from build123d import *

# Parameters (mm, degrees)
ESQUISSE1_R             = 1
BOSS_EXTRU_1_DEPTH      = 10
ESQUISSE2_W             = 4
ESQUISSE2_H             = 7.5
ESQUISSE2_H_2           = 4.5
ENL_V_MAT_EXTRU_1_DEPTH = 15


with BuildPart() as part:
    # Esquisse1 → Boss.-Extru.1 (new body)
    with BuildSketch(Plane.XY):
        with BuildLine():
            ThreePointArc((-77.855878935, 59.113903977), (-67.897166599, 55.463691844), (-64.246954466, 65.422404179))
            Line((-64.246954466, 65.422404179), (-73.709704769, 85.835790883))
            Line((-73.709704769, 85.835790883), (-75.524228032, 84.994657522))
            Line((-75.524228032, 84.994657522), (-70.47742787, 74.107517947))
            Line((-70.47742787, 74.107517947), (-74.106474395, 72.425251227))
            Line((-74.106474395, 72.425251227), (-79.153274557, 83.312390802))
            Line((-79.153274557, 83.312390802), (-81.875059451, 82.050690761))
            Line((-81.875059451, 82.050690761), (-76.828259289, 71.163551186))
            Line((-76.828259289, 71.163551186), (-80.457305814, 69.481284466))
            Line((-80.457305814, 69.481284466), (-85.504105976, 80.368424041))
            Line((-85.504105976, 80.368424041), (-87.318629238, 79.52729068))
            Line((-87.318629238, 79.52729068), (-77.855878935, 59.113903977))
        make_face()
        with Locations((-71.0514167, 62.268154078)):
            Circle(ESQUISSE1_R, mode=Mode.SUBTRACT)
    extrude(amount=BOSS_EXTRU_1_DEPTH)

    # Esquisse2 → Enlèv. mat.-Extru.1 (cut)
    with BuildSketch(Plane(origin=(-41.529278226, -19.251151014, 0), x_dir=(0, 0, 1), z_dir=(-0.9072616312569987, -0.42056668014583576, 0))):
        with BuildLine():
            Line((5, 108.875365486), (0, 108.875365486))
            Line((0, 108.875365486), (0, 103.875365486))
            ThreePointArc((0, 103.875365486), (1.464466094, 107.410899392), (5, 108.875365486))
        make_face()
        with BuildLine():
            Line((10, 108.875365486), (5, 108.875365486))
            ThreePointArc((5, 108.875365486), (8.535533906, 107.410899392), (10, 103.875365486))
            Line((10, 103.875365486), (10, 108.875365486))
        make_face()
        with BuildLine():
            ThreePointArc((6, 103.875365486), (5, 104.875365486), (4, 103.875365486))
            Line((4, 103.875365486), (6, 103.875365486))
        make_face()
        with BuildLine():
            Line((6, 103.875365486), (4, 103.875365486))
            ThreePointArc((4, 103.875365486), (5, 102.875365486), (6, 103.875365486))
        make_face()
        with Locations((5, 82.625365486)):
            Rectangle(ESQUISSE2_W, ESQUISSE2_H)
        with Locations((5, 88.625365486)):
            Rectangle(ESQUISSE2_W, ESQUISSE2_H_2)
    extrude(amount=-ENL_V_MAT_EXTRU_1_DEPTH, mode=Mode.SUBTRACT)


solid = part.part
Model file for the job. Use its own axes, mm. A direction names the side the tool comes from. Give positions to 0.01 mm unless a question says otherwise; leave off trailing zeros. Order: outer loops, then holes, each group sorted by start corner. A loop starts at its lowest first (then second) coordinate and runs counter-clockwise, first axis right, second up. Notation, with made-up numbers: (38.25, 32.25) -> (93.25, 32.25) arc R21 cw to (93.25, 42.25) -> close; hole circle Ø7 at (-7.75, 73). An arc over 180 degrees is marked (long way). Use CSV: the item, a comma, the result in double quotes.
1. Band-saw the part on A-A, the plane y = 58. Give the cut face in (x, z), then the cut area to 3 significant figures.
Outcome:
outline,"(-77.22, 0) -> (-64.88, 0) -> (-64.88, 3) -> (-77.22, 3) -> close; (-77.22, 7) -> (-64.88, 7) -> (-64.88, 10) -> (-77.22, 10) -> close"
area,"74.0 mm²"
2. Mould opens along Z. For faces 1 (the flat face through (-72.475, 78.418, 4.93)), 2 (the flat face through (-72, 65, 10)), 3 (the flat face through (-70, 61, 7)) say: +Z half, -Z half, draft (parallel to the pull), parting line (faces both ways), or undercut.
Outcome:
face 1,"draft"
face 2,"+Z half"
face 3,"undercut"
3. Drop flat-ended pins along their axis: pin 1 (4 mm diameter, centred on x = -83.5, z = 5.5, fed in from -Y); pin 2 (1.5 mm diameter, centred on x = -76.5, y = 82.5, fed in from -Z); pin 3 (6 mm diameter, centred on x = -66.5, z = 3, fed in from +Y); pin 4 (6 mm diameter, centred on x = -84.5, z = 4, fed in from +Y). Give the stop position or say it passes through.
Outcome:
pin 1,"y = 66.98"
pin 2,"through"
pin 3,"y = 76.75"
pin 4,"y = 82.18"
4. Drill centre lines: line 1 along Z through (x, y) = (-71.5, 58); line 2 along X through (y, z) = (73, 6); line 3 along X through (y, z) = (78.5, 3.25). Where is each one in solid material? Low to high. Write a range as from..to.
Outcome:
line 1,"0..3, 7..10"
line 2,"-84.29..-82.09, -77.68..-74.37, -72.87..-67.76"
line 3,"-86.84..-84.64, -80.23..-76.92, -72.51..-70.31"
5. Band-saw the part on B-B, the plane z = 0.75. Give the cut face in (x, y), then the cut area to 3 significant figures.
Outcome:
outline,"(-86.32, 77.38) -> (-77.86, 59.11) arc R7.5 ccw to (-64.25, 65.42) -> (-72.71, 83.69) -> (-74.53, 82.85) -> (-70.48, 74.11) -> (-74.11, 72.43) -> (-78.16, 81.17) -> (-80.88, 79.9) -> (-76.83, 71.16) -> (-80.46, 69.48) -> (-84.51, 78.22) -> close; hole circle Ø2 at (-71.05, 62.27)"
area,"310 mm²"
6. 3-axis set-ups, long thin cutter, end or side, ignore diameter. For faces 4 (the flat face through (-82.385, 73.639, 4.93)), 5 (the flat face through (-71, 61, 3)), 6 (the cylindrical face through (-83.9, 74.51, 5.13)): which of +Z, -Z, +X, -X, +Y, -Y reach the whole face in a straight line?
Outcome:
face 4,"+Z, -Z"
face 5,"+X, -Y"
face 6,"none"
7. Band-saw the part on D-D, the plane x = -78.5. Count the separate pieces of the cut face and the enclosed holes in it, then the cut area to 3 significant figures.
Outcome:
separate pieces,"2"
enclosed holes,"1"
area,"150 mm²"
8. Band-saw the part on C-C, the plane z = 4.5. Give the cut face in (x, y).
Outcome:
outline,"(-87.31, 79.5) -> (-85.58, 75.78) -> (-83.77, 76.62) -> (-85.49, 80.35) -> close; (-84.85, 74.21) -> (-79.75, 63.2) -> (-66.14, 69.51) -> (-71.24, 80.51) -> (-73.06, 79.67) -> (-70.48, 74.11) -> (-74.11, 72.43) -> (-76.69, 77.99) -> (-79.41, 76.73) -> (-76.83, 71.16) -> (-80.46, 69.48) -> (-83.04, 75.05) -> close; (-81.86, 82.03) -> (-80.14, 78.3) -> (-77.41, 79.56) -> (-79.14, 83.29) -> close; (-75.51, 84.97) -> (-73.79, 81.24) -> (-71.97, 82.09) -> (-73.7, 85.81) -> close"
